Answer from the drawing. Dimensions are ordinates in mm from the lowest x, y and z of the part. A direction names the side the tool comes from. Give positions to 0.01 mm unless a question says otherwise; leave off trailing zeros. Loops run counter-clockwise (first coordinate to the right, second up) from the corner with the lowest first, then second, coordinate; pieces in that order, holes last. Notation, with made-up numbers: (70, -30.5) - (120, -30.5) arc R27 cw to (120, -1.5) - close; hole circle Ø10 at (-6.75, 72.25). An arc over 180 degrees is marked (long way). Answer as CSV lines item,"result". Start each with the question number.
1) A cutting plane is placed at A-A (x = 5.65). Determine the outline of the cut face in (y, z), and give its area (3 significant figures).
2) Flat-ended cylindrical pins translate along their axes: pin 1 (3 mm diameter, centred on x = 52.15, y = 6, fed in from -Z); pin 2 (2.5 mm diameter, centred on x = 41.5, y = 5.5, fed in from +Z). Find the tip coordinate at first contact, or state that the pin passes through.
3) For the marked faces 4 and 5, determine the directions among +Z, -Z, +X, -X, +Y, -Y from which every point of the face is accessible in a straight line to the end or side of a thin tool.
4) A cutting plane is placed at D-D (y = 1.75). Determine the outline of the cut face in (x, z).
5) A cutting plane is placed at C-C (z = 2). Determine the outline of the cut face in (x, y), and give its area (3 significant figures).
6) For a pull along Y with two mould halves and no side action, classify the marked faces 1, 2 and 3 as pulls with the +Y half, pulls with the -Y half, needs draft (parallel to the pull), parting line crosses it, or undercut.
7) A cutting plane is placed at B-B (y = 6.75). Determine the outline of the cut face in (x, z), and give its area (3 significant figures).
8) Find the intervals of material crossed by line 1 along Y through (x, z) = (5.65, 3.25); line 2 along X through (y, z) = (10.25, 9); line 3 along X through (y, z) = (3, 11.25), in increasing order.
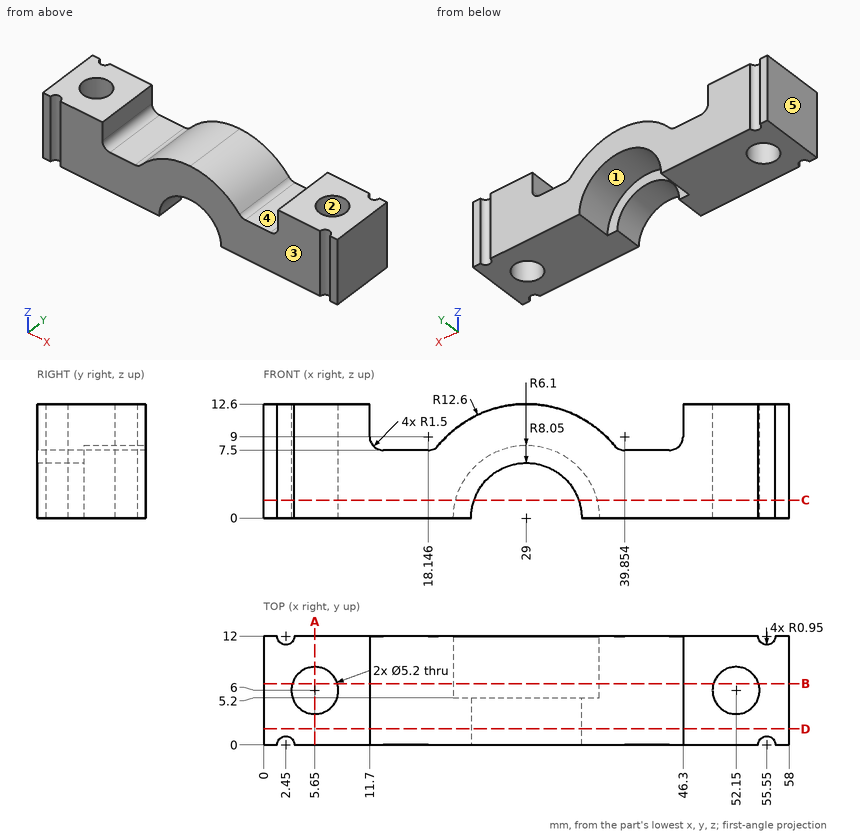
Ans:
1,outline,"(0, 0) - (3.4, 0) - (3.4, 12.6) - (0, 12.6) - close; (8.6, 0) - (12, 0) - (12, 12.6) - (8.6, 12.6) - close"
1,area,"85.7 mm2"
2,pin 1,"through"
2,pin 2,"z = 7.5"
3,face 4,"+Z, +Y, -Y"
3,face 5,"+Z, -Z, -X, +Y, -Y"
4,outline,"(0, 0) - (22.9, 0) arc R6.1 cw to (35.1, 0) - (58, 0) - (58, 12.6) - (46.3, 12.6) - (46.3, 9) arc R1.5 cw to (44.8, 7.5) - (39.85, 7.5) arc R1.5 cw to (38.7, 8.04) arc R12.6 ccw to (29, 12.6) arc R12.6 ccw to (19.3, 8.04) arc R1.5 cw to (18.15, 7.5) - (13.2, 7.5) arc R1.5 cw to (11.7, 9) - (11.7, 12.6) - (0, 12.6) - close"
5,outline,"(0, 0) - (1.5, 0) arc R0.95 cw to (3.4, 0) - (23.24, 0) - (23.24, 5.2) - (21.2, 5.2) - (21.2, 12) - (3.4, 12) arc R0.95 cw to (1.5, 12) - (0, 12) - close; (34.76, 0) - (54.6, 0) arc R0.95 cw to (56.5, 0) - (58, 0) - (58, 12) - (56.5, 12) arc R0.95 cw to (54.6, 12) - (36.8, 12) - (36.8, 5.2) - (34.76, 5.2) - close; hole circle Ø5.2 at (5.65, 6); hole circle Ø5.2 at (52.15, 6)"
5,area,"482 mm2"
6,face 1,"needs draft"
6,face 2,"undercut"
6,face 3,"pulls with the -Y half"
7,outline,"(0, 0) - (3.16, 0) - (3.16, 12.6) - (0, 12.6) - close; (8.14, 0) - (20.95, 0) arc R8.05 cw to (37.05, 0) - (49.66, 0) - (49.66, 12.6) - (46.3, 12.6) - (46.3, 9) arc R1.5 cw to (44.8, 7.5) - (39.85, 7.5) arc R1.5 cw to (38.7, 8.04) arc R12.6 ccw to (29, 12.6) arc R12.6 ccw to (19.3, 8.04) arc R1.5 cw to (18.15, 7.5) - (13.2, 7.5) arc R1.5 cw to (11.7, 9) - (11.7, 12.6) - (8.14, 12.6) - close; (54.64, 0) - (58, 0) - (58, 12.6) - (54.64, 12.6) - close"
7,area,"400 mm2"
8,line 1,"0 to 3.4, 8.6 to 12"
8,line 2,"0 to 11.7, 20.18 to 37.82, 46.3 to 58"
8,line 3,"0 to 11.7, 23.33 to 34.67, 46.3 to 58"
